```python
from build123d import *

# Parameters (mm, degrees)
SKETCH_1_W          = 28.9
SKETCH_1_H          = 186
EXTRUDE_1_DEPTH     = 3
FILLET_1_R          = 3
SKETCH_2_R          = 1.5
CUT_EXTRUDE_1_DEPTH = 3
CHAMFER_1_SIZE      = 1.5
SKETCH_3_W          = 10
SKETCH_3_H          = 30
CUT_EXTRUDE_2_DEPTH = 3
FILLET_2_R          = 3


with BuildPart() as part:
    # 草图1 → 凸台-拉伸1 (new body)
    with BuildSketch(Plane(origin=(0, 0, 0), x_dir=(1, 0, 0), z_dir=(0, 1, 0))):
        Rectangle(SKETCH_1_W, SKETCH_1_H)
    extrude(amount=EXTRUDE_1_DEPTH)

    # 圆角1
    fillet_1_edges = [part.edges().sort_by_distance(p)[0] for p in [
        (14.45, 1.5, 93),
        (-14.45, 1.5, 93),
        (-14.45, 1.5, -93),
        (14.45, 1.5, -93),
    ]]
    fillet(fillet_1_edges, radius=FILLET_1_R)

    # 草图2 → 切除-拉伸1 (cut)
    with BuildSketch(Plane(origin=(0, 3, 0), x_dir=(1, 0, 0), z_dir=(0, 1, 0))):
        with Locations(Location((-10, -89.5, 0), (0, 0, 270))):
            Circle(SKETCH_2_R)
        with Locations(Location((10, -89.5, 0), (0, 0, 90))):
            Circle(SKETCH_2_R)
        with Locations(Location((10, 89.5, 0), (0, 0, 270))):
            Circle(SKETCH_2_R)
        with Locations(Location((-10, 89.5, 0), (0, 0, 90))):
            Circle(SKETCH_2_R)
        with Locations(Location((-5, -38, 0), (0, 0, 270))):
            Circle(SKETCH_2_R)
        with Locations(Location((-5, -62, 0), (0, 0, 270))):
            Circle(SKETCH_2_R)
        with Locations(Location((5, -38, 0), (0, 0, 90))):
            Circle(SKETCH_2_R)
        with Locations(Location((5, -62, 0), (0, 0, 90))):
            Circle(SKETCH_2_R)
        with Locations(Location((5, 62, 0), (0, 0, 270))):
            Circle(SKETCH_2_R)
        with Locations(Location((5, 38, 0), (0, 0, 270))):
            Circle(SKETCH_2_R)
        with Locations(Location((-5, 62, 0), (0, 0, 90))):
            Circle(SKETCH_2_R)
        with Locations(Location((-5, 38, 0), (0, 0, 90))):
            Circle(SKETCH_2_R)
        with Locations(Location((-7.45, -7, 0), (0, 0, 270))):
            Circle(SKETCH_2_R)
        with Locations(Location((-7.45, 7, 0), (0, 0, 90))):
            Circle(SKETCH_2_R)
        with Locations(Location((10.95, 25, 0), (0, 0, 270))):
            Circle(SKETCH_2_R)
        with Locations(Location((10.95, -25, 0), (0, 0, 90))):
            Circle(SKETCH_2_R)
        with Locations(Location((-10.95, -25, 0), (0, 0, 270))):
            Circle(SKETCH_2_R)
        with Locations(Location((-10.95, 25, 0), (0, 0, 90))):
            Circle(SKETCH_2_R)
    extrude(amount=-CUT_EXTRUDE_1_DEPTH, mode=Mode.SUBTRACT)

    # 倒角1
    chamfer_1_edges = [part.edges().sort_by_distance(p)[0] for p in [
        (-7.45, 0, 5.5),
        (-5, 0, -36.5),
        (-5, 0, -60.5),
        (5, 0, -39.5),
        (-7.45, 0, -5.5),
        (10.95, 0, -26.5),
        (10.95, 0, 26.5),
        (-10.95, 0, 23.5),
        (10, 0, 91),
        (10, 0, -91),
        (-10, 0, -88),
        (-5, 0, 36.5),
        (5, 0, -63.5),
        (5, 0, 63.5),
        (5, 0, 39.5),
        (-5, 0, 60.5),
        (-10.95, 0, -23.5),
        (-10, 0, 88),
    ]]
    chamfer(chamfer_1_edges, length=CHAMFER_1_SIZE)

    # 草图3 → 切除-拉伸2 (cut)
    with BuildSketch(Plane(origin=(0, 3, 0), x_dir=(1, 0, 0), z_dir=(0, 1, 0))):
        with Locations((4.45, 0)):
            Rectangle(SKETCH_3_W, SKETCH_3_H)
    extrude(amount=-CUT_EXTRUDE_2_DEPTH, mode=Mode.SUBTRACT)

    # 圆角2
    fillet_2_edges = [part.edges().sort_by_distance(p)[0] for p in [
        (9.45, 1.5, -15),
        (9.45, 1.5, 15),
        (-0.55, 1.5, 15),
        (-0.55, 1.5, -15),
    ]]
    fillet(fillet_2_edges, radius=FILLET_2_R)


solid = part.part
```
Read the model definition and answer for the solid it produces. Units are mm, in the model's axes. A direction names the side the tool comes from. Coordinates: 2 decimals unless noted, no trailing zeros. Answer as a JSON object with one key per item and string values.
Q1. Determine the mould class of faces 1 (the flat face through (-3, 0, -1)), 2 (the cylindrical face through (5.9, 2.3, 39.2)), 3 (the flat face through (14.45, 1, 1)) for opening direction X: pulls with the +X half, pulls with the -X half, needs draft (parallel to the pull), parting line crosses it, or undercut.
The answers:
{"face 1": "needs draft", "face 2": "undercut", "face 3": "pulls with the +X half"}
Q2. A tool of negligible diameter and unlimited length cuts with its end or side. For faces 4 (the cylindrical face through (-13.59, 1.52, -92.1)), 5 (the cylindrical face through (0.35, 1.48, -14.14)), from which of +Z, -Z, +X, -X, +Y, -Y can it reach the whole face along a straight path? Write none if from no direction.
The answers:
{"face 4": "-Z, -X, +Y, -Y", "face 5": "+Y, -Y"}
Q3. The part is cut by section A-A on y = 2.2. Give the number of separate pieces and of enclosed holes in the cut face, then the cut area to 3 significant figures.
The answers:
{"separate pieces": "1", "enclosed holes": "19", "area": "4,950 mm2"}
Q4. Flat-ended cylindrical pins translate along their axes: pin 1 Ø1.8 at (x, z) = (-10.95, -25) entering from -Y; pin 2 Ø3.5 at (x, z) = (-5, -62) entering from -Y. Find the tip coordinate at first contact, or state that the pin passes through.
The answers:
{"pin 1": "passes through", "pin 2": "stops at y = 1.25"}
Q5. Consider line 1 (X direction, y = 2.85, z = -38); line 2 (X direction, y = 2.05, z = 25); line 3 (Z direction, x = 12.25, y = 1.1). Determine where each line is inside the solid, lowest interval first. Write a range as [from, to].
The answers:
{"line 1": "x = [-14.45, -6.5], [-3.5, 3.5], [6.5, 14.45]", "line 2": "x = [-14.45, -12.45], [-9.45, 9.45], [12.45, 14.45]", "line 3": "z = [-92.89, -26.39], [-23.61, 23.61], [26.39, 92.89]"}
